Input: dimensioned drawing with shaded views. Units: mm. Origin: part minimum x, y, z. A direction names the side the tool comes from. Coordinates: 2 decimals unless noted, no trailing zeros. Order: outer loops, then holes, each group sorted by start corner. A loop starts at its lowest first (then second) coordinate and runs counter-clockwise, first axis right, second up. Notation, with made-up numbers: M 68.5,76 L 125.5,76 A14 ccw 125.5,99 Z; hole C -0.5,47.5 d2. An arc over 180 degrees is marked long. Write item = value, one per line.
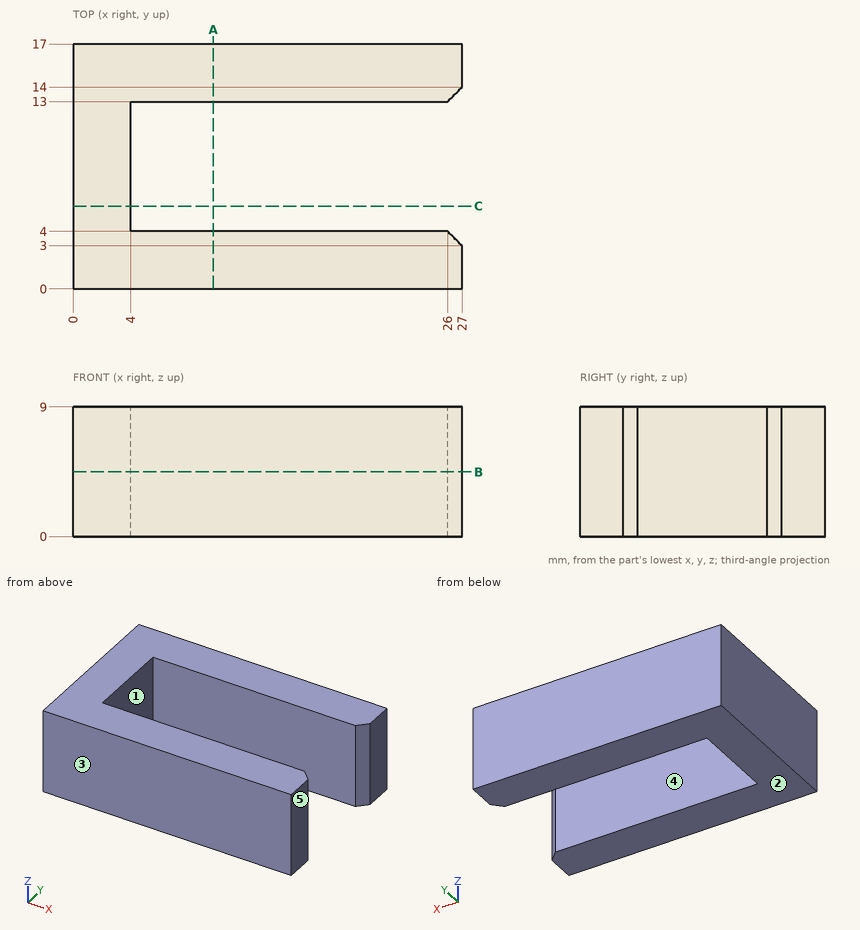
1) Mould query, pull axis Y, two halves, no side actions, for the marked faces 1, 2 and 3. Classes: pulls with the +Y half, pulls with the -Y half, needs draft (parallel to the pull), parting line crosses it, or undercut.
Numbers:
face_1 = undercut
face_2 = needs draft
face_3 = pulls with the -Y half
2) Section B-B, the plane z = 4.5. Return loops of the section in (x, y), and give its area (3 significant figures).
Numbers:
outline = M 0,0 L 27,0 L 27,3 L 26,4 L 4,4 L 4,13 L 26,13 L 27,14 L 27,17 L 0,17 Z
area = 251 mm²
3) Line query: L1, parallel to Y at x = 7, z = 6.75; L2, parallel to X at y = 10, z = 0.5; L3, parallel to Y at x = 26.25, z = 4. Output: solid intervals per line, ascending.
Numbers:
L1 = 0 to 4, 13 to 17
L2 = 0 to 4
L3 = 0 to 3.75, 13.25 to 17
4) Section C-C, the plane y = 5.75. Return loops of the section in (x, z).
Numbers:
outline = M 0,0 L 4,0 L 4,9 L 0,9 Z
5) Set-up query: the marked faces 4 and 5. Return all of +Z, -Z, +X, -X, +Y, -Y with unobstructed straight access to the full face (end or side cutting, diameter ignored); none if empty.
Numbers:
face_4 = +Z, -Z, +X
face_5 = +Z, -Z, +X, +Y, -Y
6) Section A-A, the plane x = 9.75. Return loops of the section in (y, z).
Numbers:
outline = M 0,0 L 4,0 L 4,9 L 0,9 Z; M 13,0 L 17,0 L 17,9 L 13,9 Z
7) Pin query (flat end, axial travel): pin 1 (6 mm diameter, centred on x = 11.5, y = 14.5, fed in from -Z). Return the tip coordinate at first contact, or that it passes through.
Numbers:
pin_1 = 0
